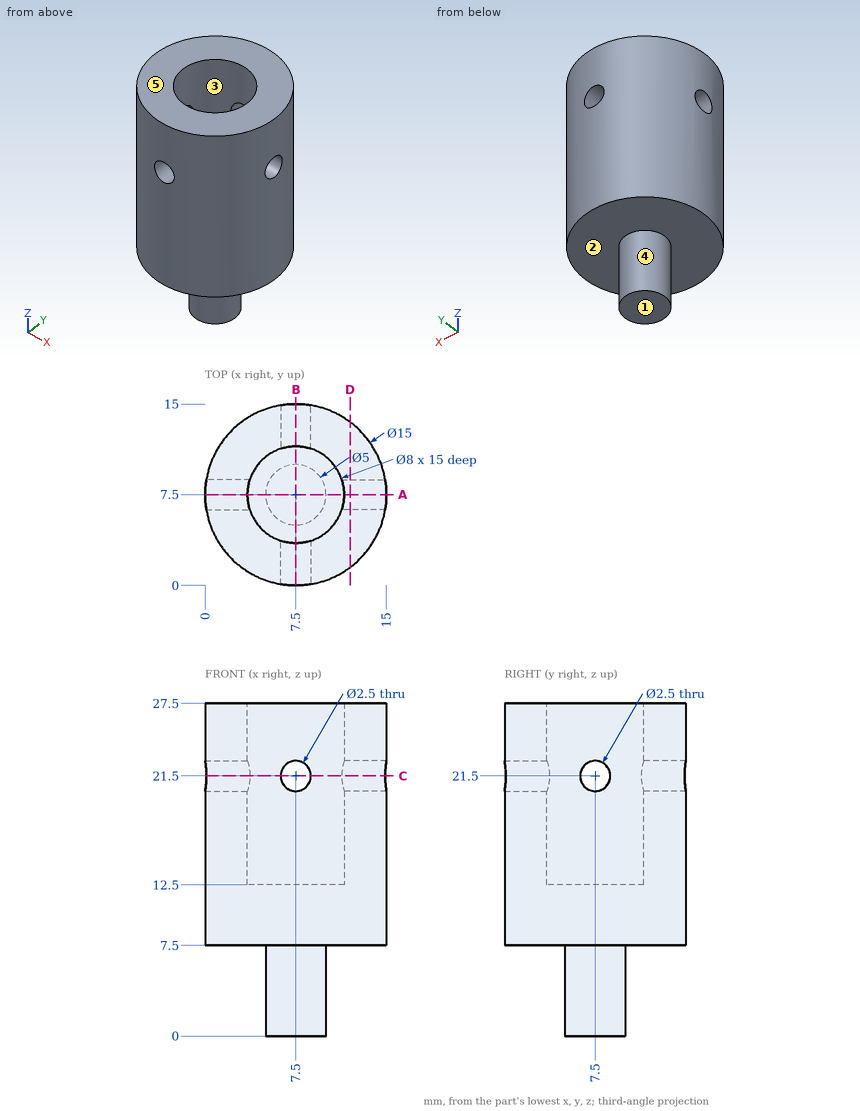
Job drawing, mm, ordinate dimensions from the low corner. One solid piece. A direction names the side the tool comes from. Give positions to 0.01 mm unless a question says otherwise; leave off trailing zeros. Write each loop counter-clockwise with the first axis right and the second up, starting at its lowest first coordinate (ties: lowest second). Pieces come first, ordered by that corner, then holes. Notation, with made-up numbers: (75.25, 43) - (91.25, 43) arc R24 ccw to (91.25, 65) - close; hole circle Ø6 at (69.25, -8.5). An arc over 180 degrees is marked (long way). Use one line per item in the form item = value. Start each with the question number.
1. Drop flat-ended pins along their axis: pin 1 Ø3 at (y, z) = (2, 23) entering from -X; pin 2 Ø3 at (y, z) = (7.5, 21.5) entering from +X; pin 3 Ø2 at (x, y) = (7.5, 13) entering from -Z. Give the stop position or say it passes through.
2. 3-axis set-ups, long thin cutter, end or side, ignore diameter. For the marked faces 1 and 2: which of +Z, -Z, +X, -X, +Y, -Y reach the whole face in a straight line?
3. Band-saw the part on C-C on z = 21.5. Write the cut outline in (x, y).
4. Band-saw the part on A-A on y = 7.5. Write the cut outline in (x, z), plus the area to 3 significant figures.
5. Band-saw the part on D-D on x = 12. Write the cut outline in (y, z), plus the area to 3 significant figures.
6. Two-plate mould, pull along Y, no slides. Class the marked faces 3, 4 and 5: released by +Y, released by -Y, zero draft, split by the parting line, or undercut.
7. Probe line 1 (Z direction, x = 7.5, y = 12.25); line 2 (Y direction, x = 10.75, z = 20.5); line 3 (Y direction, x = 4.75, z = 22.5). List the from-to ranges inside material, lowest first. Write a range as [from, to].
Conclusion:
q1.pin_1 = 1.16
q1.pin_2 = 15
q1.pin_3 = 7.5
q2.face_1 = -Z, +X, -X, +Y, -Y
q2.face_2 = -Z
q3.outline = (0.1, 6.25) arc R7.5 ccw to (6.25, 0.1) - (6.25, 3.7) arc R4 cw to (3.7, 6.25) - close; (0.1, 8.75) - (3.7, 8.75) arc R4 cw to (6.25, 11.3) - (6.25, 14.9) arc R7.5 ccw to start; (8.75, 0.1) arc R7.5 ccw to (14.9, 6.25) - (11.3, 6.25) arc R4 cw to (8.75, 3.7) - close; (8.75, 11.3) arc R4 cw to (11.3, 8.75) - (14.9, 8.75) arc R7.5 ccw to (8.75, 14.9) - close
q4.outline = (0, 7.5) - (5, 7.5) - (5, 0) - (10, 0) - (10, 7.5) - (15, 7.5) - (15, 20.25) - (11.5, 20.25) - (11.5, 12.5) - (3.5, 12.5) - (3.5, 20.25) - (0, 20.25) - close; (0, 22.75) - (3.5, 22.75) - (3.5, 27.5) - (0, 27.5) - close; (11.5, 22.75) - (15, 22.75) - (15, 27.5) - (11.5, 27.5) - close
q4.area = 200 mm²
q5.outline = (1.5, 7.5) - (13.5, 7.5) - (13.5, 27.5) - (1.5, 27.5) - close; hole circle Ø2.5 at (7.5, 21.5)
q5.area = 235 mm²
q6.face_3 = undercut
q6.face_4 = split by the parting line
q6.face_5 = zero draft
q7.line_1 = [7.5, 20.25], [22.75, 27.5]
q7.line_2 = [0.74, 5.17], [9.83, 14.26]
q7.line_3 = [0.52, 4.6], [10.4, 14.48]
